Geometry check sheet. Reference: the model listing, model coordinates, mm. Face numbers are marked on the shaded views. A direction names the side the tool comes from. Give positions to 0.01 mm unless a question says otherwise; leave off trailing zeros. Write each loop counter-clockwise with the first axis right and the second up, starting at its lowest first coordinate (ties: lowest second). Pieces come first, ordered by that corner, then holes. Notation, with made-up numbers: (53, -35) - (74, -35) arc R11 ccw to (74, -30) - close; hole circle Ø2 at (-3.75, 65). An arc over 180 degrees is marked (long way). One line per question, with ' | ' between items. Start each with the question number.
Q1. Thickness scan on L1, parallel to Y at x = 36, z = 12; L2, parallel to X at y = 37, z = -6.5; L3, parallel to Z at x = 67.5, y = 55. Record the ranges inside material, lowest first. Write a range as [from, to].
Q2. Release check for a two-part mould opening along Y. For the marked faces 4, 5 and 6 record: +Y half, -Y half, draft (parallel to the pull), parting line (faces both ways), or undercut.
Q3. Set-up check for the marked faces 1, 2 and 3: record each of +Z, -Z, +X, -X, +Y, -Y from which the full face is reachable in a straight line by a thin tool's end or side.
Q4. Section check B-B on y = 32. Record the boundary of the cut face in (x, z).
Q5. Section check D-D on y = 54. Record the boundary of the cut face in (x, z), and give its area (3 significant figures).
Q6. Gauge pin test, flat ends, axial feed: P1, Ø12, axis at x = 56.5, y = 27, coming from the -Z side; P2, Ø5, axis at x = 137.5, y = 33.5, coming from the +Z side; P3, Ø5.5, axis at x = 36, y = 10, coming from the +Z side. Record the tip position at first contact, or that the pin passes through.
Q7. Section check A-A on x = 83. Record the boundary of the cut face in (y, z), and give its area (3 significant figures).
Q8. Section check C-C on z = -9. Record the boundary of the cut face in (x, y), and give its area (3 significant figures).
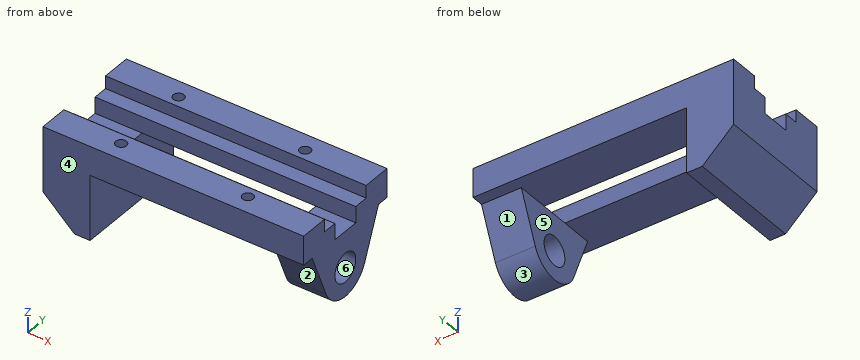
```python
from build123d import *

# Parameters (mm, degrees)
BOSS_EXTRUDE2_DEPTH     = 64
SKETCH8_R               = 8
BOSS_EXTRUDE3_DEPTH     = 22
CUT_EXTRUDE1_DEPTH      = 162.641578809
CUT_EXTRUDE1_DEPTH_BACK = 162.641578809
SKETCH9_R               = 3
CUT_EXTRUDE2_DEPTH      = 11


with BuildPart() as part:
    # Sketch3 → Boss-Extrude2 (new body)
    with BuildSketch(Plane(origin=(0, 0, 0), x_dir=(1, 0, 0), z_dir=(0, 1, 0))):
        Polygon((26, 36), (26, 0), (144, 0), (144, -16), (0, -16), (0, 0), (0, 20), (17.362220716, 36), align=None)
    extrude(amount=BOSS_EXTRUDE2_DEPTH)

    # Sketch8 → Boss-Extrude3 (add)
    with BuildSketch(Plane(origin=(144, 0, 0), x_dir=(0, 0, -1), z_dir=(1, 0, 0))):
        with BuildLine():
            Line((0, 57.460004127), (0, 6.539995873))
            Line((0, 6.539995873), (26.053796804, 17.189478596))
            ThreePointArc((26.053796804, 17.189478596), (36, 32), (26.053796804, 46.810521404))
            Line((26.053796804, 46.810521404), (0, 57.460004127))
        make_face()
        with Locations((20, 32)):
            Circle(SKETCH8_R, mode=Mode.SUBTRACT)
    extrude(amount=-BOSS_EXTRUDE3_DEPTH)

    # Sketch8_6 → Cut-Extrude1 (cut, two sides: drawn at the far end of the back side and taken through both)
    with BuildSketch(Plane(origin=(144, 0, 0), x_dir=(0, 0, -1), z_dir=(1, 0, 0)).offset(-CUT_EXTRUDE1_DEPTH_BACK)):
        Polygon((0, 24), (0, 40), (-9, 40), (-9, 48), (-16, 48), (-16, 32), (-16, 16), (-9, 16), (-9, 24), align=None)
    extrude(amount=CUT_EXTRUDE1_DEPTH + CUT_EXTRUDE1_DEPTH_BACK, mode=Mode.SUBTRACT)

    # Sketch9 → Cut-Extrude2 (cut)
    with BuildSketch(Plane.XY.offset(16)):
        with Locations((106, 54)):
            Circle(SKETCH9_R)
        with Locations((36, 10)):
            Circle(SKETCH9_R)
        with Locations((106, 10)):
            Circle(SKETCH9_R)
        with Locations((36.080551107, 54)):
            Circle(SKETCH9_R)
    extrude(amount=-CUT_EXTRUDE2_DEPTH, mode=Mode.SUBTRACT)


solid = part.part
```
Working result:
1) L1: y = [0, 7], [13, 16], [48, 51], [57, 64] | L2: x = [0, 26], [122, 144] | L3: z = [0, 16]
2) face 4: -Y half | face 5: draft | face 6: undercut
3) face 1: -Z, +X, +Y | face 2: -Z, +X, -Y | face 3: -Z, +X
4) outline: (0, -20) - (17.36, -36) - (26, -36) - (26, 0) - (0, 0) - close; (122, -36) - (144, -36) - (144, -28) - (122, -28) - close; (122, -12) - (144, -12) - (144, 0) - (122, 0) - close
5) outline: (0, -20) - (17.36, -36) - (26, -36) - (26, 0) - (122, 0) - (122, -8.46) - (144, -8.46) - (144, 16) - (109, 16) - (109, 5) - (103, 5) - (103, 16) - (39.08, 16) - (39.08, 5) - (33.08, 5) - (33.08, 16) - (0, 16) - close | area: 3,160 mm2
6) P1: stops at z = 0 | P2: stops at z = 0 | P3: stops at z = 5
7) outline: (0, 0) - (24, 0) - (24, 9) - (16, 9) - (16, 16) - (0, 16) - close; (40, 0) - (64, 0) - (64, 16) - (48, 16) - (48, 9) - (40, 9) - close | area: 656 mm2
8) outline: (0, 0) - (26, 0) - (26, 64) - (0, 64) - close; (122, 10.22) - (144, 10.22) - (144, 53.78) - (122, 53.78) - close | area: 2,620 mm2
